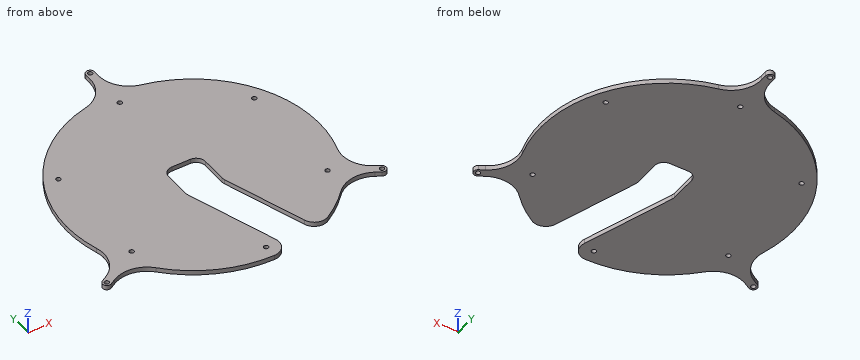
from build123d import *

# Parameters (mm, degrees)
SKETCH1_R           = 82.5
SKETCH1_R_2         = 1.5
BOSS_EXTRUDE1_DEPTH = 3
CUT_EXTRUDE1_DEPTH  = 117.711181984
FILLET1_R           = 6
BOSS_EXTRUDE2_START = -3
SKETCH3_R           = 1.5
BOSS_EXTRUDE2_DEPTH = 3
CIRPATTERN1_COUNT   = 3


with BuildPart() as part:
    # Sketch1 → Boss-Extrude1 (new body)
    with BuildSketch(Plane.XY):
        Circle(SKETCH1_R)
        with Locations((0, 74)):
            Circle(SKETCH1_R_2, mode=Mode.SUBTRACT)
        with Locations((0, -74)):
            Circle(SKETCH1_R_2, mode=Mode.SUBTRACT)
        with Locations((64.08587988, 37)):
            Circle(SKETCH1_R_2, mode=Mode.SUBTRACT)
        with Locations((64.08587988, -37)):
            Circle(SKETCH1_R_2, mode=Mode.SUBTRACT)
        with Locations((-64.08587988, -37)):
            Circle(SKETCH1_R_2, mode=Mode.SUBTRACT)
        with Locations((-64.08587988, 37)):
            Circle(SKETCH1_R_2, mode=Mode.SUBTRACT)
    extrude(amount=BOSS_EXTRUDE1_DEPTH)

    # Sketch2 → Cut-Extrude1 (cut, through all)
    with BuildSketch(Plane.XY.offset(3)):
        with BuildLine():
            Line((12, -12), (30.275351929, -66.024842017))
            ThreePointArc((30.275351929, -66.024842017), (35.411833596, -71.285530901), (42.729580876, -70.572182325))
            ThreePointArc((42.729580876, -70.572182325), (22.181579725, -79.462113746), (0, -82.5))
            ThreePointArc((0, -82.5), (6.906581307, -78.954708332), (8.051787281, -71.276266978))
            Line((8.051787281, -71.276266978), (-12, -12))
            Line((-12, -12), (-12, 12))
            Line((-12, 12), (12, 12))
            Line((12, 12), (12, -12))
        make_face()
    extrude(amount=-CUT_EXTRUDE1_DEPTH, mode=Mode.SUBTRACT)

    # Fillet1
    fillet1_edges = [part.edges().sort_by_distance(p)[0] for p in [
        (12, 12, 1.5),
        (12, -12, 1.5),
        (-12, -12, 1.5),
        (-12, 12, 1.5),
    ]]
    fillet(fillet1_edges, radius=FILLET1_R)

    # Sketch3 → Boss-Extrude2 (add)
    with BuildSketch(Plane.XY.offset(3).offset(BOSS_EXTRUDE2_START)):
        with BuildLine():
            Line((2.75, 104), (2.75, 99.943421494))
            ThreePointArc((2.75, 99.943421494), (7.117014236, 87.469057539), (18.31097561, 80.442266081))
            ThreePointArc((18.31097561, 80.442266081), (0, 82.5), (-18.31097561, 80.442266081))
            ThreePointArc((-18.31097561, 80.442266081), (-7.117014236, 87.469057539), (-2.75, 99.943421494))
            Line((-2.75, 99.943421494), (-2.75, 104))
            ThreePointArc((-2.75, 104), (0, 106.75), (2.75, 104))
        make_face()
        with Locations((0, 104)):
            Circle(SKETCH3_R, mode=Mode.SUBTRACT)
    boss_extrude2 = extrude(amount=BOSS_EXTRUDE2_DEPTH)

    # CirPattern1: Boss-Extrude2 ×3 about axis
    cirpattern1_axis = Axis((0, 0, 0), (0, 0, 1))
    for i in range(1, CIRPATTERN1_COUNT):
        add(boss_extrude2.rotate(cirpattern1_axis, i * 360 / CIRPATTERN1_COUNT))


solid = part.part
Here's how the part is built. I have some questions about the finished solid (model axes, mm). Coordinates: 2 decimals unless noted, no trailing zeros. Loops run counter-clockwise (first coordinate to the right, second up) from the corner with the lowest first, then second, coordinate; pieces in that order, holes last. Notation, with made-up numbers: (-32, 44.25) -> (-27, 44.25) arc R26 cw to (-27, 74.25) -> close; hole circle Ø11 at (-1.5, -38.75). An arc over 180 degrees is marked (long way). Use one line per item in the form item = value. Start each with the question number.
(1) Please list where these lines run through material, in increasing order: line 1 along X through (y, z) = (104, 1.85); line 2 along X through (y, z) = (-67, 0.9); line 3 along Y through (x, z) = (-64.5, 1.05).
(2) If we section it at A-A (x = -50): Please give me the cut outline in (y, z).
(3) Will these pins go through, and if not, where does the flat tip stop? pin 1 (0.9 mm diameter, centred on y = 102, z = 1.5, fed in from -X); pin 2 (3.5 mm diameter, centred on x = -64.09, y = 37, fed in from +Z); pin 3 (1.5 mm diameter, centred on x = 2, z = 1, fed in from -Y); pin 4 (1.5 mm diameter, centred on y = -1, z = 2, fed in from +X).
(4) If we section it at C-C (y = 23): Please give me the cut outline in (x, z), then the cut area to 3 significant figures.
(5) If we section it at B-B (z = 2.2): Give the number of separate pieces and of enclosed holes in the cut face, then the cut area to 3 significant figures.
Verdict:
q1.line_1 = -2.75 to -1.5, 1.5 to 2.75
q1.line_2 = -48.14 to 6.61, 30.67 to 48.14
q1.line_3 = -52.76 to -38.44, -35.56 to 35.56, 38.44 to 51.44
q2.outline = (-65.62, 0) -> (65.62, 0) -> (65.62, 3) -> (-65.62, 3) -> close
q3.pin_1 = -2.75
q3.pin_2 = 3
q3.pin_3 = -82.41
q3.pin_4 = 82.5
q4.outline = (-79.23, 0) -> (79.23, 0) -> (79.23, 3) -> (-79.23, 3) -> close
q4.area = 475 mm²
q5.separate_pieces = 1
q5.enclosed_holes = 9
q5.area = 19,800 mm²
